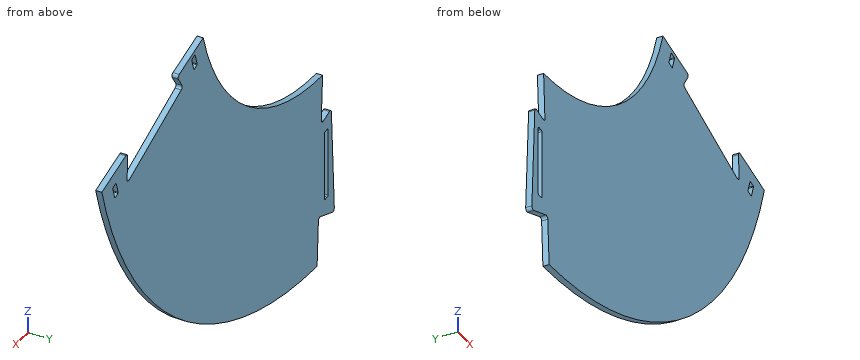
Autodesk Inventor part; units mm, degrees
ref_plane "YZ Plane" through (0, 0, 0) normal (1, 0, 0) x (0, 1, 0)
ref_plane "XZ Plane" through (0, 0, 0) normal (0, 1, 0) x (-1, 0, 0)
ref_plane "XY Plane" through (0, 0, 0) normal (0, 0, 1) x (1, 0, 0)
sketch "Sketch1" plane through (0, 0, 0) normal (0, 1, 0) x (-1, 0, 0)
  circle A0 centre (0, 0) radius 425
  circle A1 centre (0, 0) radius 233.71
  dimension "d84" = 467.42
  dimension "d85" = 850
extrude "Extrusion3" add sketch "Sketch1" along normal blind 6
sketch "Sketch2" plane through (0, 6, 0) normal (0, 1, 0) x (1, 0, 0)
  circle A0 centre (0, 0) radius 329.355 construction
  line L0 (3.25, 363.0217) -> (3.25, 295.6883)
  line L1 (-3.25, 295.6883) -> (-3.25, 363.0217)
  arc A1 (-3.25, 295.6883) -> (-1.9167, 294.355) centre (-1.9167, 295.6883) ccw
  arc A2 (1.9167, 294.355) -> (3.25, 295.6883) centre (1.9167, 295.6883) ccw
  arc A3 (-1.9167, 364.355) -> (-3.25, 363.0217) centre (-1.9167, 363.0217) ccw
  arc A4 (3.25, 363.0217) -> (1.9167, 364.355) centre (1.9167, 363.0217) ccw
  line L2 (-1.9167, 364.355) -> (1.9167, 364.355)
  line L3 (-1.9167, 294.355) -> (1.9167, 294.355)
  line L4 (0, 294.355) -> (0, 329.355) construction
  line L5 (0, 364.355) -> (0, 329.355) construction
  line L6 (0, 364.355) -> (0, 294.355) construction
  line L7 (175.0629, -238.5433) -> (171.9617, -240.7965)
  arc A5 (176.9253, -238.8383) -> (175.0629, -238.5433) centre (175.8467, -239.622) ccw
  arc A6 (171.9617, -240.7965) -> (171.6667, -242.6589) centre (172.7454, -241.8752) ccw
  line L8 (173.0175, -238.1382) -> (193.59, -266.4538) construction
  line L9 (211.2443, -297.1327) -> (171.6667, -242.6589)
  line L10 (176.9253, -238.8383) -> (216.5029, -293.3121)
  line L11 (214.1625, -294.7694) -> (173.0175, -238.1382) construction
  line L12 (214.1625, -294.7694) -> (193.59, -266.4538) construction
  arc A7 (211.2443, -297.1327) -> (213.1067, -297.4277) centre (212.323, -296.349) ccw
  line L13 (216.2079, -295.1745) -> (213.1067, -297.4277)
  arc A8 (216.2079, -295.1745) -> (216.5029, -293.3121) centre (215.4242, -294.0958) ccw
  line L14 (280.1548, 92.2019) -> (281.3393, 88.5562)
  arc A9 (281.0108, 93.882) -> (280.1548, 92.2019) centre (281.4229, 92.614) ccw
  arc A10 (281.3393, 88.5562) -> (283.0194, 87.7002) centre (282.6074, 88.9682) ccw
  line L15 (279.9482, 90.9607) -> (313.2352, 101.7763) construction
  line L16 (347.0573, 108.5073) -> (283.0194, 87.7002)
  line L17 (281.0108, 93.882) -> (345.0486, 114.6892)
  line L18 (346.5222, 112.5919) -> (279.9482, 90.9607) construction
  line L19 (346.5222, 112.5919) -> (313.2352, 101.7763) construction
  arc A11 (347.0573, 108.5073) -> (347.9133, 110.1874) centre (346.6452, 109.7754) ccw
  line L20 (346.7287, 113.8331) -> (347.9133, 110.1874)
  arc A12 (346.7287, 113.8331) -> (345.0486, 114.6892) centre (345.4607, 113.4211) ccw
  dimension "d86" = 658.71
  dimension "d21" = 6.5
  dimension "d24" = 2.6667
  dimension "d25" = 2.6667
  dimension "d32" = 1.3333
  dimension "d33" = 1.3333
  dimension "d162" = 70
  dimension "d163" = 294.355
  dimension "d165" = 3.25
extrude "Extrusion4" cut sketch "Sketch2" against normal through all
sketch "Sketch3" plane through (0, 6, 0) normal (0, 1, 0) x (1, 0, 0)
  arc A0 (-131.3389, -404.1968) -> (131.3445, -404.195) centre (0, 0) ccw
  arc A1 (-77.7244, -128.3741) -> (77.7297, -128.3709) centre (0, 0) ccw
  line L0 (-122.1811, -173.696) -> (-161.3589, -227.6196)
  line L1 (-131.3389, -404.1968) -> (-77.7244, -128.3741)
  line L2 (0, 0) -> (0, -341.2918)
  line L3 (131.3445, -404.195) -> (77.7297, -128.3709)
  line L4 (210.5535, -295.3313) -> (171.3679, -241.3969)
  dimension "d52" = 25
  dimension "d87" = 150.07
  dimension "d88" = 425
  dimension "d89" = 25
  dimension "d90" = 11
  dimension "d91" = 11
sketch "Sketch5" plane through (0, 6, 0) normal (0, 1, 0) x (1, 0, 0)
  line L0 (3.25, 363.0217) -> (3.25, 295.6883)
  line L1 (5.5862, 281.6788) -> (-6.155, 278.5328)
  line L2 (-11.2263, 385.43) -> (10.5847, 377.0575)
  line L3 (6.5657, 233.6709) -> (8.9394, 278.9635)
  line L4 (14.2034, 379.4075) -> (16.5771, 424.7001)
  arc A0 (10.5847, 377.0575) -> (14.2034, 379.4075) centre (11.5404, 379.5471) ccw
  arc A1 (8.9394, 278.9635) -> (5.5862, 281.6788) centre (6.2763, 279.103) ccw
  arc A2 (-11.2263, 385.43) -> (-14.8449, 382.8009) centre (-12.1819, 382.9405) ccw
  line L5 (-3.25, 295.6883) -> (-3.25, 363.0217)
  line L6 (-14.8449, 382.8009) -> (-9.5081, 280.969)
  arc A3 (-9.5081, 280.969) -> (-6.155, 278.5328) centre (-6.8451, 281.1086) ccw
  line L7 (-1.9167, 294.355) -> (1.9167, 294.355)
  line L8 (1.9167, 364.355) -> (-1.9167, 364.355)
  line L9 (16.5771, 424.7001) -> (16.5774, 424.7058)
  line L10 (6.5657, 233.6709) -> (6.5621, 233.6028)
  circle A4 centre (0, 0) radius 425
  circle A5 centre (0, 0) radius 233.71
  line L11 (-356.4489, 130.7516) -> (-398.7912, 147.0053)
  arc A6 (-355.3322, 126.5839) -> (-356.4489, 130.7516) centre (-357.4046, 128.2621) ccw
  line L12 (-370.0348, 108.4276) -> (-355.3322, 126.5839)
  arc A7 (-370.0348, 108.4276) -> (-368.6526, 104.1736) centre (-367.9624, 106.7494) ccw
  line L13 (-368.6526, 104.1736) -> (-270.1556, 77.7814)
  arc A8 (-270.1556, 77.7814) -> (-266.8024, 80.2177) centre (-269.4654, 80.3572) ccw
  line L14 (-266.1663, 92.3563) -> (-266.8024, 80.2177)
  arc A9 (-262.5476, 94.7063) -> (-266.1663, 92.3563) centre (-263.5032, 92.2167) ccw
  line L15 (-220.2053, 78.4526) -> (-262.5476, 94.7063)
  line L16 (-220.2053, 78.4526) -> (-220.1417, 78.4282)
  line L17 (-398.7912, 147.0053) -> (-398.7965, 147.0073)
  line L18 (-142.66, -185.1845) -> (-142.6172, -185.1316)
  line L19 (-263.0436, -333.8458) -> (-263.0472, -333.8502)
  line L20 (132.0366, -192.9029) -> (131.9995, -192.8458)
  line L21 (236.2213, -353.3334) -> (236.2244, -353.3381)
  line L22 (365.2271, 103.7351) -> (409.0364, 115.4738)
  arc A10 (361.8739, 106.4505) -> (365.2271, 103.7351) centre (364.5369, 106.3109) ccw
  line L23 (363.0966, 129.7812) -> (361.8739, 106.4505)
  arc A11 (363.0966, 129.7812) -> (359.478, 132.4103) centre (360.4336, 129.9208) ccw
  line L24 (359.478, 132.4103) -> (264.2793, 95.867)
  arc A12 (264.2793, 95.867) -> (262.9985, 91.9251) centre (265.2349, 93.3774) ccw
  line L25 (269.6187, 81.7308) -> (262.9985, 91.9251)
  arc A13 (268.0724, 77.7026) -> (269.6187, 81.7308) centre (267.3822, 80.2784) ccw
  line L26 (224.2631, 65.9639) -> (268.0724, 77.7026)
  line L27 (224.2631, 65.9639) -> (224.1973, 65.9463)
  line L28 (409.0364, 115.4738) -> (409.0419, 115.4753)
  line L29 (0, -233.71) -> (0, -425)
  arc A14 (131.3445, -404.195) -> (-131.3389, -404.1968) centre (0, 0) ccw
  point P0 (-425, 0)
  point P1 (-425, 0)
  point P2 (-398.7693, 146.9969)
  point P3 (-220.1557, 78.4336)
  point P4 (16.5759, 424.6766)
  point P5 (6.5629, 233.6178)
  point P6 (409.0137, 115.4677)
  point P7 (224.2118, 65.9502)
  dimension "d63" = 2.6667
  dimension "d64" = 3
  dimension "d66" = 3
  dimension "d67" = 2.6667
  dimension "d68" = 2.6667
  dimension "d70" = 72
  dimension "d71" = 72
sketch "Sketch6" plane through (0, 6, 0) normal (0, 1, 0) x (1, 0, 0)
  line L0 (237.9351, -331.8846) -> (247.6433, -324.8312)
  line L1 (243.8227, -319.5725) -> (234.1145, -326.626)
  line L2 (210.5535, -295.3313) -> (171.3679, -241.3969)
  line L3 (215.5172, -293.3731) -> (212.416, -295.6263)
  arc A0 (244.7539, -319.72) -> (243.8227, -319.5725) centre (244.2145, -320.1119) ccw
  arc A1 (247.6433, -324.8312) -> (247.7908, -323.9) centre (247.2514, -324.2918) ccw
  arc A2 (237.0039, -331.7371) -> (237.9351, -331.8846) centre (237.5432, -331.3452) ccw
  arc A3 (234.1145, -326.626) -> (233.967, -327.5572) centre (234.5063, -327.1653) ccw
  line L4 (233.967, -327.5572) -> (237.0039, -331.7371)
  line L5 (247.7908, -323.9) -> (244.7539, -319.72)
  line L6 (171.3679, -241.3969) -> (210.5535, -295.3313)
  line L7 (190.9607, -268.3641) -> (196.2193, -264.5435)
  line L8 (215.8122, -291.5107) -> (176.6265, -237.5763)
  line L9 (145.065, -204.0599) -> (154.7732, -197.0065)
  line L10 (158.5938, -202.2651) -> (148.8856, -209.3185)
  arc A4 (158.5938, -202.2651) -> (158.7413, -201.3339) centre (158.202, -201.7257) ccw
  arc A5 (155.7044, -197.154) -> (154.7732, -197.0065) centre (155.1651, -197.5458) ccw
  arc A6 (145.065, -204.0599) -> (144.9175, -204.9911) centre (145.4569, -204.5992) ccw
  arc A7 (147.9544, -209.171) -> (148.8856, -209.3185) centre (148.4938, -208.7792) ccw
  line L11 (147.9544, -209.171) -> (144.9175, -204.9911)
  line L12 (155.7044, -197.154) -> (158.7413, -201.3339)
  point P0 (0, 0)
  dimension "d104" = 6.5
  dimension "d105" = 12
  dimension "d108" = 1.3333
  dimension "d109" = 1.3333
  dimension "d110" = 1.3333
  dimension "d111" = 1.3333
  dimension "d112" = 0
  dimension "d149" = 145
  dimension "d150" = 90
  dimension "d151" = 90
  dimension "d152" = 90
  dimension "d153" = 90
extrude "Extrusion7" cut sketch "Sketch6" against normal through all
pattern_circular "Circular Pattern2" count 2 over 72 about axis through (0, -10, 0) along (0, 1, 0) of "Extrusion7"
pattern_circular "Circular Pattern3" count 2 over 144 about axis through (0, -10, 0) along (0, 1, 0) of "Extrusion7"
mirror "Mirror3" about plane through (0, 0, 0) normal (1, 0, 0) of "Extrusion7"
extrude "Extrusion10" cut sketch "Sketch3" against normal blind 10
mirror "Mirror4" about plane through (0, 0, 0) normal (1, 0, 0) of "Extrusion4"
pattern_circular "Circular Pattern4" count 2 over 144 about axis through (0, -10, 0) along (0, -1, 0) of "Extrusion7"
extrude "Extrusion11" cut sketch "Sketch5" against normal through all contours A1 L3 L10 A5 L16 L15 A9 L14 A8 L13 A7 L12 A6 L11 A4 L4 A0 L2 A2 L6 A3 L1 | L27 L26 A13 L25 A12 L24 A11 L23 A10 L22 A4 L29 A5 | A5 L29 A4 L11 A6 L12 A7 L13 A8 L14 A9 L15 L16
equation "\"BendRadius\" = Thickness"
equation "\"BendReliefWidth\" = Thickness"
equation "\"BendReliefDepth\" = 0.5 * Thickness"
equation "\"CornerReliefSize\" = 4 * Thickness"
equation "\"MinimumRemnant\" = 2 * Thickness"
equation "\"TransitionRadius\" = BendRadius"
equation "\"JacobiRadiusSize\" = BendRadius"
equation "\"GapSize\" = Thickness"
properties part number "Ring C3" material "Wood (Maple)"
Check sheet for the modelled part. Datum: model origin and axes. Units: mm. Coordinates: 2 decimals unless noted, no trailing zeros. Write each loop counter-clockwise with the first axis right and the second up, starting at its lowest first coordinate (ties: lowest second). Pieces come first, ordered by that corner, then holes. Notation, with made-up numbers: M 2.25,2.25 L 23.25,2.25 A15 ccw 23.25,8.25 Z; hole C 70,-4 d7. An arc over 180 degrees is marked long. Write item = value, one per line. Start each with the question number.
1. Sectioned sample at A-A (z = -356). Record the cut outline in (x, y).
2. Go/stop test with flat-tipped pins: pin 1 (1.8 mm diameter, centred on y = 2, z = -337.5, fed in from +X); pin 2 (3 mm diameter, centred on y = 2.5, z = -321.5, fed in from -X); pin 3 (3 mm diameter, centred on x = 0.5, y = 2, fed in from -Z). Record where each tip stops, or that it passes through.
3. Sectioned sample at C-C (z = -306.5). Record the cut outline in (x, y).
4. Sectioned sample at D-D (x = 282.5). Record the cut outline in (y, z).
5. Thickness scan on probe 1 along X at (y, z) = (5.65, -341.5); probe 2 along X at (y, z) = (4.95, -86); probe 3 along X at (y, z) = (0.3, -238). Record the ranges inside material, lowest first.
6. Sectioned sample at B-B (y = 4.6). State how many separate pieces and enclosed holes the cut face has, then the cut area to 3 significant figures.
The answers:
q1.outline = M -13.44,0 L -3.25,0 L -3.25,6 L -13.44,6 Z; M 3.25,0 L 232.14,0 L 232.14,6 L 3.25,6 Z
q2.pin_1 = 259.47
q2.pin_2 = -11.71
q2.pin_3 = -381.5
q3.outline = M -10.85,0 L -3.25,0 L -3.25,6 L -10.85,6 Z; M 3.25,0 L 294.42,0 L 294.42,6 L 3.25,6 Z
q4.outline = M 0,-317.52 L 6,-317.52 L 6,-102.86 L 0,-102.86 Z
q5.probe_1 = -12.68 to -3.25, 3.25 to 252.99
q5.probe_2 = 217.31 to 235.3, 242.13 to 266.85
q5.probe_3 = 6.79 to 352.11
q6.separate_pieces = 1
q6.enclosed_holes = 3
q6.area = 78,500 mm²
